Geometry check sheet. Reference: the model listing, model coordinates, mm. Give positions to 0.01 mm unless a question says otherwise; leave off trailing zeros. Order: outer loops, then holes, each group sorted by start corner. A loop starts at its lowest first (then second) coordinate and runs counter-clockwise, first axis right, second up. Notation, with made-up numbers: M -24,48.25 L 16,48.25 A27 ccw 16,83.25 Z; hole C 10.25,33 d6. An arc over 180 degrees is marked long. Answer as CSV lines item,"result".
from build123d import *

# Parameters (mm, degrees)
SCHIZZO1_R                   = 2.5
SCHIZZO1_W                   = 10
SCHIZZO1_H                   = 2.5
ESTRUSIONE_ESTRUSIONE1_DEPTH = 2


with BuildPart() as part:
    # Schizzo1 → Estrusione-Estrusione1 (new body)
    with BuildSketch(Plane(origin=(0, 0, 0), x_dir=(0, 0, -1), z_dir=(1, 0, 0))):
        with BuildLine():
            Line((80, -7.5), (-80, -7.5))
            ThreePointArc((-80, -7.5), (-87.5, 0), (-80, 7.5))
            Line((-80, 7.5), (80, 7.5))
            ThreePointArc((80, 7.5), (87.5, 0), (80, -7.5))
        make_face()
        with Locations((-80, 0)):
            Circle(SCHIZZO1_R, mode=Mode.SUBTRACT)
        with Locations((80, 0)):
            Circle(SCHIZZO1_R, mode=Mode.SUBTRACT)
        with Locations((-10, 0)):
            Circle(SCHIZZO1_R, mode=Mode.SUBTRACT)
        with Locations((15, 0)):
            Rectangle(SCHIZZO1_W, SCHIZZO1_H, mode=Mode.SUBTRACT)
        with Locations((55, 0)):
            Rectangle(SCHIZZO1_W, SCHIZZO1_H, mode=Mode.SUBTRACT)
    extrude(amount=ESTRUSIONE_ESTRUSIONE1_DEPTH)


solid = part.part
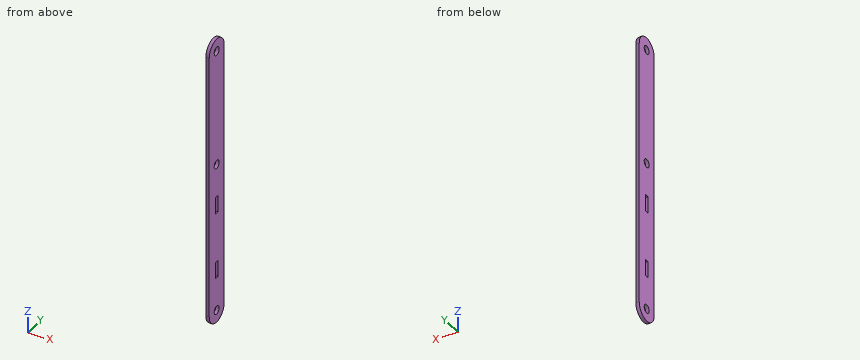
(1) Section check B-B on z = -14.5. Enter the section's corners in (x, y), then the cut area to 3 significant figures.
The answers:
outline,"M 0,-7.5 L 2,-7.5 L 2,-1.25 L 0,-1.25 Z; M 0,1.25 L 2,1.25 L 2,7.5 L 0,7.5 Z"
area,"25.0 mm2"
(2) Section check C-C on y = -6. Enter the section's corners in (x, z), then the cut area to 3 significant figures.
The answers:
outline,"M 0,-84.5 L 2,-84.5 L 2,84.5 L 0,84.5 Z"
area,"338 mm2"
(3) Section check A-A on x = 0.75. Enter the section's corners in (y, z).
The answers:
outline,"M -7.5,-80 A7.5 ccw 7.5,-80 L 7.5,80 A7.5 ccw -7.5,80 Z; hole C 0,-80 d5; hole C 0,10 d5; hole C 0,80 d5; hole M -1.25,-60 L 1.25,-60 L 1.25,-50 L -1.25,-50 Z; hole M -1.25,-20 L 1.25,-20 L 1.25,-10 L -1.25,-10 Z"
(4) Material ranges on line 1 (Y direction, x = 0.65, z = -80); line 2 (Z direction, x = 1, y = 1.5); line 3 (Z direction, x = 1.6, y = -4), recorded low to high.
The answers:
line 1,"y = -7.5 to -2.5, 2.5 to 7.5"
line 2,"z = -87.35 to -82, -78 to 8, 12 to 78, 82 to 87.35"
line 3,"z = -86.34 to 86.34"
(5) Gauge pin test, flat ends, axial feed: P1, Ø1, axis at x = 1, y = 6, coming from the -Z side; P2, Ø0.6, axis at x = 1, y = 0.5, coming from the -Z side. Record the tip position at first contact, or that the pin passes through.
The answers:
P1,"stops at z = -85.1"
P2,"stops at z = -87.5"
